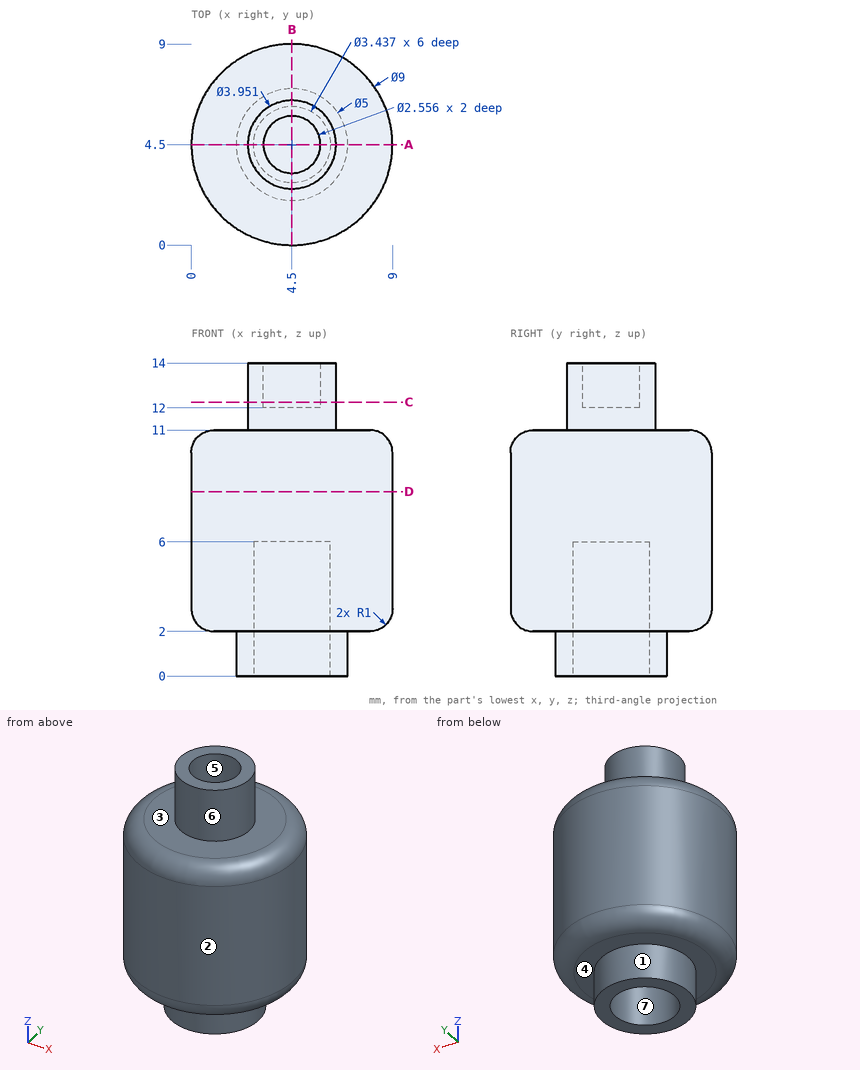
The drawing under review shows one solid part. Ordinate dimensions are in mm from its lowest x, y, z. A direction names the side the tool comes from. Coordinates: 2 decimals unless noted, no trailing zeros. Write each loop counter-clockwise with the first axis right and the second up, starting at its lowest first coordinate (ties: lowest second). Pieces come first, ordered by that corner, then holes. Notation, with made-up numbers: (12.25, 8.5) -> (47.25, 8.5) arc R23 ccw to (47.25, 29.5) -> close; hole circle Ø2 at (-24.75, -29). An arc over 180 degrees is marked (long way). One line per item, written item: value. Start each with the question number.
Q1. Add section D-D, the plane z = 8.25. Give the boundary of the cut face in (x, y), then the cut area to 3 significant figures.
Q2. Clearance check with flat-ended pins moving along their axes: P1, Ø1, axis at x = 5, y = 4.5, coming from the -Z side; P2, Ø2, axis at y = 6.5, z = 1.5, coming from the -X side (1 decimal); P3, Ø2, axis at x = 4.5, z = 12.5, coming from the -Y side. State where each tip first meets the part, or that it passes through.
Q3. For the marked faces 1, 2 and 3, list the 3-axis set-ups (+Z, -Z, +X, -X, +Y, -Y) from which the entire face can be reached by the end or side of a thin tool; tool diameter is ignored.
Q4. Add section C-C, the plane z = 12.25. Give the boundary of the cut face in (x, y) (1 decimal).
Q5. To check wall thickness, follow probe 1 along Y at (x, z) = (4.5, 1.3); probe 2 along Y at (x, z) = (4.5, 13.15) (1 decimal); probe 3 along Z at (x, y) = (6.5, 3.5). State the ranges of each line that lie inside material, in increasing order.
Q6. The part is to be moulded in two halves that separate along Y. For the marked faces 4, 5, 6 and 7, say which applies: +Y half, -Y half, draft (parallel to the pull), parting line (faces both ways), or undercut.
Q7. Add section A-A, the plane y = 4.5. Give the boundary of the cut face in (x, z) (1 decimal).
Response:
1. outline: circle Ø9 at (4.5, 4.5)
1. area: 63.6 mm²
2. P1: z = 6
2. P2: x = 0.5
2. P3: y = 2.52
3. face 1: -Z
3. face 2: +Z, -Z
3. face 3: +Z
4. outline: circle Ø4 at (4.5, 4.5); hole circle Ø2.6 at (4.5, 4.5)
5. probe 1: 2 to 2.78, 6.22 to 7
5. probe 2: 2.5 to 3.2, 5.8 to 6.5
5. probe 3: 0 to 11
6. face 4: draft
6. face 5: undercut
6. face 6: parting line
6. face 7: undercut
7. outline: (0, 3) arc R1 ccw to (1, 2) -> (2, 2) -> (2, 0) -> (2.8, 0) -> (2.8, 6) -> (6.2, 6) -> (6.2, 0) -> (7, 0) -> (7, 2) -> (8, 2) arc R1 ccw to (9, 3) -> (9, 10) arc R1 ccw to (8, 11) -> (6.5, 11) -> (6.5, 14) -> (5.8, 14) -> (5.8, 12) -> (3.2, 12) -> (3.2, 14) -> (2.5, 14) -> (2.5, 11) -> (1, 11) arc R1 ccw to (0, 10) -> close
